from build123d import *

# Parameters (mm, degrees)
BOSS_EXTRUDE1_DEPTH      = 40
BOSS_EXTRUDE2_DEPTH      = 1
BOSS_EXTRUDE2_DEPTH_BACK = 3
CUT_EXTRUDE1_DEPTH       = 73.740978822
SKETCH5_R                = 1.75
CUT_EXTRUDE2_DEPTH       = 73.740978822
FILLET1_R                = 2
CUT_EXTRUDE3_REACH       = 76.935
SKETCH6_R                = 1.75


# Read off the part's stored shape, not the designer's step: moBlkMgr[Ga_GB37]
with BuildPart() as part:
    # Sketch1 → Boss-Extrude1 (new body)
    with BuildSketch(Plane(origin=(0, 0, 0), x_dir=(1, 0, 0), z_dir=(0, 1, 0))):
        Polygon((0, 0), (0, 27), (3, 27), (3, 3), (42.5, 3), (42.5, 0), align=None)
    extrude(amount=BOSS_EXTRUDE1_DEPTH)

    # Sketch2 → Boss-Extrude2 (add, two sides: drawn at the far end of the back side and taken through both)
    with BuildSketch(Plane(origin=(3, 0, 0), x_dir=(0, 0, -1), z_dir=(1, 0, 0)).offset(-BOSS_EXTRUDE2_DEPTH_BACK)):
        with BuildLine():
            Line((3, 0), (27, 0))
            ThreePointArc((27, 0), (47, 20), (27, 40))
            Line((27, 40), (3, 40))
            Line((3, 40), (3, 0))
        make_face()
    extrude(amount=BOSS_EXTRUDE2_DEPTH + BOSS_EXTRUDE2_DEPTH_BACK)

    # Sketch3 → Cut-Extrude1 (cut, through all)
    with BuildSketch(Plane(origin=(4, 0, 0), x_dir=(0, 0, -1), z_dir=(1, 0, 0))):
        with BuildLine():
            Line((20, 26.5), (34, 26.5))
            ThreePointArc((34, 26.5), (40.5, 20), (34, 13.5))
            Line((34, 13.5), (20, 13.5))
            ThreePointArc((20, 13.5), (13.5, 20), (20, 26.5))
        make_face()
    extrude(amount=-CUT_EXTRUDE1_DEPTH, mode=Mode.SUBTRACT)

    # Sketch5 → Cut-Extrude2 (cut, through all)
    with BuildSketch(Plane(origin=(4, 0, 0), x_dir=(0, 0, -1), z_dir=(1, 0, 0))):
        with Locations((27, 4.5)):
            Circle(SKETCH5_R)
        with Locations((13.576606241, 12.25)):
            Circle(SKETCH5_R)
        with Locations((13.576606241, 27.75)):
            Circle(SKETCH5_R)
        with Locations((27, 35.5)):
            Circle(SKETCH5_R)
        with Locations((40.423393759, 27.75)):
            Circle(SKETCH5_R)
        with Locations((40.423393759, 12.25)):
            Circle(SKETCH5_R)
    extrude(amount=-CUT_EXTRUDE2_DEPTH, mode=Mode.SUBTRACT)

    # Fillet1
    fillet1_edges = [part.edges().sort_by_distance(p)[0] for p in [
        (0, 20, 0),
        (42.5, 0, -1.5),
        (42.5, 40, -1.5),
    ]]
    fillet(fillet1_edges, radius=FILLET1_R)

    # Sketch6 → Cut-Extrude3 (cut, up to next)
    with BuildSketch(Plane.XY, mode=Mode.PRIVATE) as cut_extrude3_sk1:
        with Locations((34.5, 5)):
            Circle(SKETCH6_R)
    cut_extrude3_tool1 = extrude(cut_extrude3_sk1.sketch, amount=-CUT_EXTRUDE3_REACH, mode=Mode.PRIVATE) & part.part
    # Sketch6 → Cut-Extrude3 (cut, up to next)
    with BuildSketch(Plane.XY, mode=Mode.PRIVATE) as cut_extrude3_sk2:
        with Locations((34.5, 35)):
            Circle(SKETCH6_R)
    cut_extrude3_tool2 = extrude(cut_extrude3_sk2.sketch, amount=-CUT_EXTRUDE3_REACH, mode=Mode.PRIVATE) & part.part
    # Sketch6 → Cut-Extrude3 (cut, up to next)
    with BuildSketch(Plane.XY, mode=Mode.PRIVATE) as cut_extrude3_sk3:
        with Locations((10.5, 35)):
            Circle(SKETCH6_R)
    cut_extrude3_tool3 = extrude(cut_extrude3_sk3.sketch, amount=-CUT_EXTRUDE3_REACH, mode=Mode.PRIVATE) & part.part
    # Sketch6 → Cut-Extrude3 (cut, up to next)
    with BuildSketch(Plane.XY, mode=Mode.PRIVATE) as cut_extrude3_sk4:
        with Locations((10.5, 5)):
            Circle(SKETCH6_R)
    cut_extrude3_tool4 = extrude(cut_extrude3_sk4.sketch, amount=-CUT_EXTRUDE3_REACH, mode=Mode.PRIVATE) & part.part
    add(cut_extrude3_tool1.solids().sort_by_distance((34.5, 5, 0))[0], mode=Mode.SUBTRACT)
    add(cut_extrude3_tool2.solids().sort_by_distance((34.5, 35, 0))[0], mode=Mode.SUBTRACT)
    add(cut_extrude3_tool3.solids().sort_by_distance((10.5, 35, 0))[0], mode=Mode.SUBTRACT)
    add(cut_extrude3_tool4.solids().sort_by_distance((10.5, 5, 0))[0], mode=Mode.SUBTRACT)


solid = part.part
Work out the finished part from the listing and answer in its coordinate system (mm). A direction names the side the tool comes from. Round coordinates to 2 decimals unless told otherwise and drop trailing zeros. Order: outer loops, then holes, each group sorted by start corner. A loop starts at its lowest first (then second) coordinate and runs counter-clockwise, first axis right, second up. Notation, with made-up numbers: M 10,-20 L 20,-20 A14 cw 20,-10 Z; hole C -3.75,-18 d11. An arc over 180 degrees is marked long. Put each result on its own line as item: value. Start each with the question number.
Q1. Section A-A, the plane x = 10.5 is taken. Write down the section's boundary in (y, z).
Q2. Flat-ended cylindrical pins translate along their axes: pin 1 (4.5 mm diameter, centred on x = 1.5, z = -24.5, fed in from -Y); pin 2 (10 mm diameter, centred on x = 18, y = 12, fed in from -Z); pin 3 (10 mm diameter, centred on y = 32.5, z = -16.5, fed in from +X). Find the tip coordinate at first contact, or state that the pin passes through.
Q3. Section D-D, the plane y = 18 is taken. Write down the section's boundary in (x, z), and give its area (3 significant figures).
Q4. Section C-C, the plane y = 27.75 is taken. Write down the section's boundary in (x, z), and give its area (3 significant figures).
Q5. For a pull along Z with two mould halves and no side action, classify faces 4 (the flat face through (23, 20, -3)), 5 (the flat face through (2, 13.5, -27)), 6 (the flat face through (11.3, 40, -2.6)), 7 (the cylindrical face through (2.03, 27.08, -42.04)) as pulls with the +Z half, pulls with the -Z half, needs draft (parallel to the pull), parting line crosses it, or undercut.
Q6. Straight lines are drawn through the part: L1, parallel to Y at x = 10.5, z = -2.25; L2, parallel to Z at x = 15, y = 38; L3, parallel to X at y = 29, z = -16. For each, find the intervals that lie inside material, in ascending order. Write a range as [from, to].
Q7. Section B-B, the plane z = -29.5 is taken. Write down the section's boundary in (x, y), and give its area (3 significant figures).
Q8. A tool of negligible diameter and unlimited length cuts with its end or side. For faces 1 (the flat face through (4, 25, -15)), 2 (the cylindrical face through (2, 19.9, -13.5)), 3 (the cylindrical face through (11.31, 33.45, -1.48)), from which of +Z, -Z, +X, -X, +Y, -Y can it reach the whole face along a straight path? Write none if from no direction.
Findings below:
1. outline: M 0,-3 L 3.25,-3 L 3.25,0 L 0,0 Z; M 6.75,-3 L 33.25,-3 L 33.25,0 L 6.75,0 Z; M 36.75,-3 L 40,-3 L 40,0 L 36.75,0 Z
2. pin 1: stops at y = 0
2. pin 2: stops at z = -3
2. pin 3: stops at x = 4
3. outline: M 0,-46.9 L 4,-46.9 L 4,-40.18 L 0,-40.18 Z; M 0,-13.82 L 4,-13.82 L 4,-3 L 42.5,-3 L 42.5,0 L 2,0 A2 ccw 0,-2 Z
3. area: 197 mm^2
4. outline: M 0,-45.44 L 4,-45.44 L 4,-42.17 L 0,-42.17 Z; M 0,-38.67 L 4,-38.67 L 4,-15.33 L 0,-15.33 Z; M 0,-11.83 L 4,-11.83 L 4,-3 L 42.5,-3 L 42.5,0 L 2,0 A2 ccw 0,-2 Z
4. area: 268 mm^2
5. face 4: pulls with the -Z half
5. face 5: undercut
5. face 6: needs draft
5. face 7: undercut
6. L1: y = [0, 3.25], [6.75, 33.25], [36.75, 40]
6. L2: z = [-3, 0]
6. L3: x = [0, 4]
7. outline: M 0,0.16 L 4,0.16 L 4,13.5 L 0,13.5 Z; M 0,26.5 L 4,26.5 L 4,39.84 L 0,39.84 Z
7. area: 107 mm^2
8. face 1: -Z, +X, +Y, -Y
8. face 2: +X, -X
8. face 3: +Z, -Z
